Source: three-view drawing plus pictorial views. Frame: mm from the lowest corner of the part. Give positions to 0.01 mm unless a question says otherwise; leave off trailing zeros. Loops run counter-clockwise (first coordinate to the right, second up) from the corner with the lowest first, then second, coordinate; pieces in that order, holes last. Notation, with made-up numbers: M 53.25,82 L 88.25,82 A17 cw 88.25,104 Z; hole C 3.5,9.25 d4. An arc over 180 degrees is marked long. Answer as a JSON object with one key per item and string values. Group by question number.
1) Section query B-B on z = 0.3. Count the separate pieces of the cut face and the enclosed holes in it, plus the area to 3 significant figures.
2) Section query D-D on x = 4. Return loops of the section in (y, z), plus the area to 3 significant figures.
3) Section query A-A on y = 26.33. Return loops of the section in (x, z).
4) Section query C-C on y = 30. Return loops of the section in (x, z), plus the area to 3 significant figures.
5) Ray query, L1, parallel to X at y = 18.71, z = 0.2; L2, parallel to X at y = 11.5, z = 0.2; L3, parallel to X at y = 2, z = 0.6. Return the intervals inside material, ascending.
6) First-contact query: P1, Ø1.9, axis at x = 3, y = 31.2, coming from the -Z side; P2, Ø8, axis at x = 6.5, y = 20, coming from the -Z side. Flat tips, straight axial feed; report the tip coordinate or a pass-through.
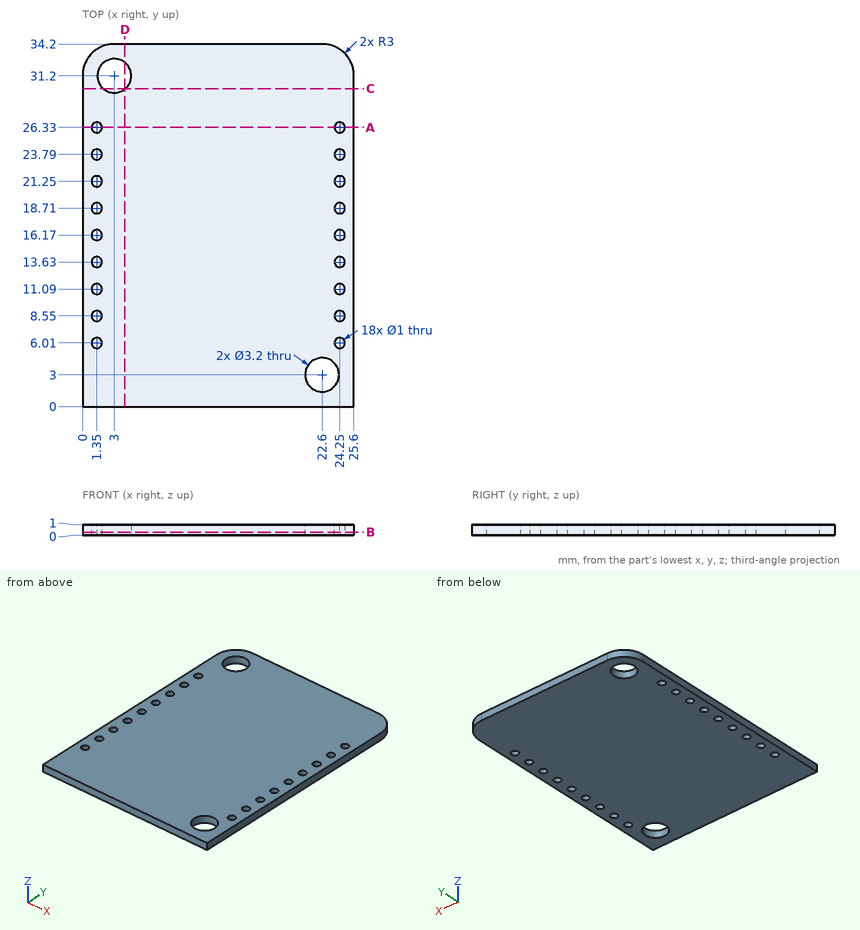
Output:
{
 "1": {"separate pieces": "1", "enclosed holes": "20", "area": "841 mm^2"},
 "2": {"outline": "M 0,0 L 29.95,0 L 29.95,1 L 0,1 Z; M 32.45,0 L 34.2,0 L 34.2,1 L 32.45,1 Z", "area": "31.7 mm^2"},
 "3": {"outline": "M 0,0 L 0.85,0 L 0.85,1 L 0,1 Z; M 1.85,0 L 23.75,0 L 23.75,1 L 1.85,1 Z; M 24.75,0 L 25.6,0 L 25.6,1 L 24.75,1 Z"},
 "4": {"outline": "M 0,0 L 1.94,0 L 1.94,1 L 0,1 Z; M 4.06,0 L 25.6,0 L 25.6,1 L 4.06,1 Z", "area": "23.5 mm^2"},
 "5": {"L1": "x = 0 to 0.85, 1.85 to 23.75, 24.75 to 25.6", "L2": "x = 0 to 1.06, 1.64 to 23.96, 24.54 to 25.6", "L3": "x = 0 to 21.35, 23.85 to 25.6"},
 "6": {"P1": "passes through", "P2": "stops at z = 0"}
}
